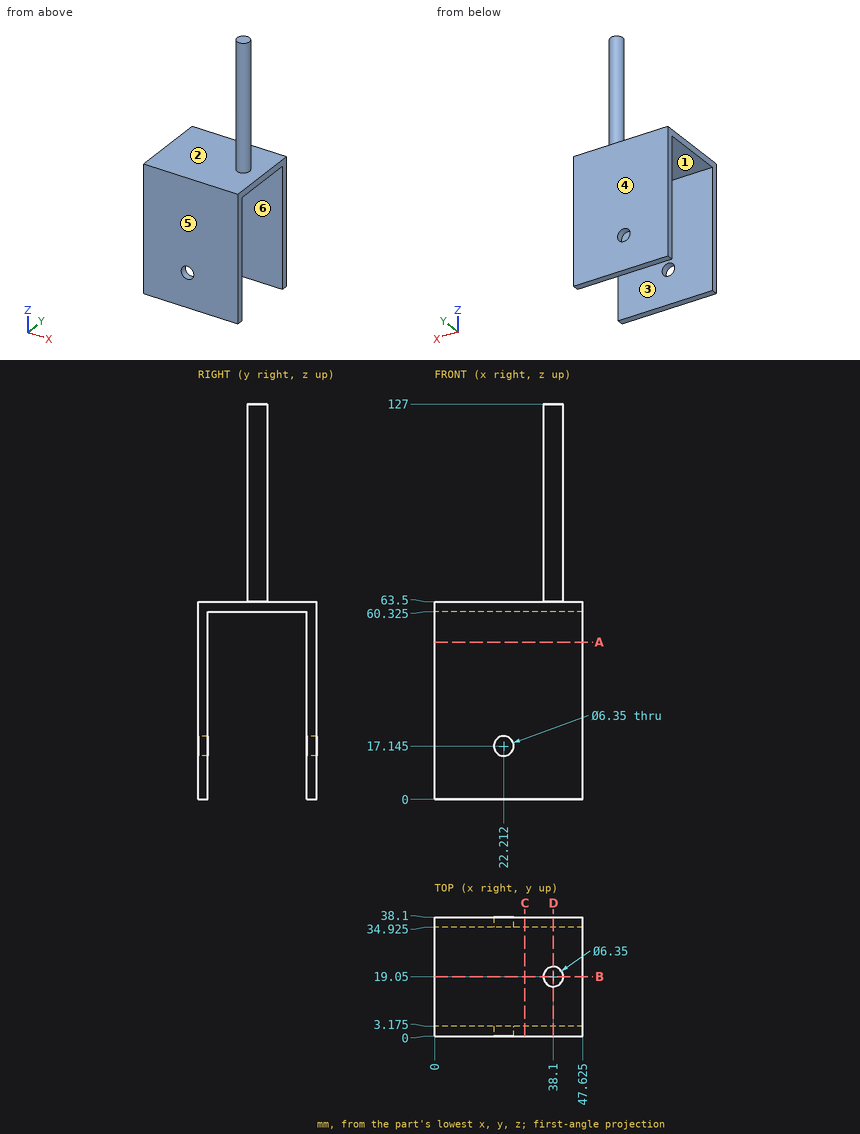
Could you check a few things on this drawing? It's one solid part, dimensions in mm from its lowest x, y, z. A direction names the side the tool comes from. Coordinates: 2 decimals unless noted, no trailing zeros. Order: outer loops, then holes, each group sorted by start corner. A loop starts at its lowest first (then second) coordinate and runs counter-clockwise, first axis right, second up. Notation, with made-up numbers: (6.5, -2.5) - (34.5, -2.5) arc R19 ccw to (34.5, 22.5) - close; hole circle Ø10 at (-36, 47). An arc over 180 degrees is marked (long way). Answer as a JSON object with one key per item and string values. Group by question number.
Q1. Imagine slicing it at D-D (x = 38.1). Please give me the cut outline in (y, z) (3 decimals), and give its area (3 significant figures).
Q2. We'd pull the mould along Y, two halves only. Please class the marked faces 1, 2, 3 and 4: +Y half, -Y half, draft (parallel to the pull), parting line (faces both ways), or undercut.
Q3. On a 3-axis mill with a long thin cutter (end or side, diameter ignored), from which of +Z, -Z, +X, -X, +Y, -Y can I reach the whole of each face in a straight line? I mean the marked faces 5 and 6. Say none if no direction works.
Q4. Will these pins go through, and if not, where does the flat tip stop? P1, Ø6, axis at x = 21.5, y = 18, coming from the -Z side (3 decimals); P2, Ø11.5, axis at x = 14, y = 27.5, coming from the +Z side; P3, Ø5, axis at y = 17, z = 105.5, coming from the -X side (3 decimals).
Q5. Imagine slicing it at C-C (x = 29). Please give me the cut outline in (y, z) (3 decimals).
Q6. Imagine slicing it at A-A (z = 50.5). Please give me the cut outline in (x, y) (3 decimals), and give its area (3 significant figures).
Q7. I need wall thicknesses on line 1 (Y direction, x = 17.5, z = 50) (3 decimals); line 2 (Z direction, x = 35.5, y = 33.5) (3 decimals); line 3 (Z direction, x = 39, y = 16.5) (3 decimals). Which ranges of each line are inside material? Lowest first, please. Write a range as from..to.
Q8. Imagine slicing it at B-B (y = 19.05). Please give me the cut outline in (x, z) (3 decimals).
Determined:
{
 "1": {"outline": "(0, 0) - (3.175, 0) - (3.175, 60.325) - (34.925, 60.325) - (34.925, 0) - (38.1, 0) - (38.1, 63.5) - (22.225, 63.5) - (22.225, 127) - (15.875, 127) - (15.875, 63.5) - (0, 63.5) - close", "area": "907 mm2"},
 "2": {"face 1": "undercut", "face 2": "draft", "face 3": "undercut", "face 4": "+Y half"},
 "3": {"face 5": "+Z, -Z, +X, -X, -Y", "face 6": "-Z, +X, -X"},
 "4": {"P1": "stops at z = 60.325", "P2": "stops at z = 63.5", "P3": "stops at x = 34.925"},
 "5": {"outline": "(0, 0) - (3.175, 0) - (3.175, 60.325) - (34.925, 60.325) - (34.925, 0) - (38.1, 0) - (38.1, 63.5) - (0, 63.5) - close"},
 "6": {"outline": "(0, 0) - (47.625, 0) - (47.625, 3.175) - (0, 3.175) - close; (0, 34.925) - (47.625, 34.925) - (47.625, 38.1) - (0, 38.1) - close", "area": "302 mm2"},
 "7": {"line 1": "y = 0..3.175, 34.925..38.1", "line 2": "z = 60.325..63.5", "line 3": "z = 60.325..127"},
 "8": {"outline": "(0, 60.325) - (47.625, 60.325) - (47.625, 63.5) - (41.275, 63.5) - (41.275, 127) - (34.925, 127) - (34.925, 63.5) - (0, 63.5) - close"}
}
